Design review of the part built by this model. Coordinates are the model's own, in mm. Face numbers are marked on the shaded views. Coordinates: 2 decimals unless noted, no trailing zeros. Order: outer loops, then holes, each group sorted by start corner. A loop starts at its lowest first (then second) coordinate and runs counter-clockwise, first axis right, second up. Notation, with made-up numbers: M 35,-18.5 L 87,-18.5 A24 ccw 87,-2.5 Z; hole C 9.5,36 d7. An arc over 180 degrees is marked long. Answer as a JSON object with one key per item and string values.
from build123d import *

# Parameters (mm, degrees)
SKETCH1_R                = 25.4
BOSS_EXTRUDE1_DEPTH      = 127
BOSS_EXTRUDE2_REACH      = 202
BOSS_EXTRUDE2_END_RADIUS = 25.4
SKETCH3_R                = 12.7
SKETCH4_R                = 20
BOSS_EXTRUDE3_DEPTH      = 12.7
FILLET1_R                = 15.08


with BuildPart() as part:
    # Sketch1 → Boss-Extrude1 (new body)
    with BuildSketch(Plane(origin=(0, 0, 0), x_dir=(1, 0, 0), z_dir=(0, 1, 0))):
        with Locations(Location((0, 0, 0), (0, 0, 270))):
            Circle(SKETCH1_R)
    extrude(amount=BOSS_EXTRUDE1_DEPTH)

    # Boss-Extrude2: up to this cylinder (the profile starts outside it)
    boss_extrude2_end = Plane(origin=(0, 19.05, 0), z_dir=(0, -1, 0)) * Cylinder(BOSS_EXTRUDE2_END_RADIUS, 455.8, mode=Mode.PRIVATE)
    # Sketch3 → Boss-Extrude2 (add, up to the surface)
    with BuildSketch(Plane(origin=(127, 0, 0), x_dir=(0, 0, -1), z_dir=(1, 0, 0)), mode=Mode.PRIVATE) as boss_extrude2_sk1:
        with Locations((0, 19.05)):
            Circle(SKETCH3_R)
    boss_extrude2_tool1 = extrude(boss_extrude2_sk1.sketch, amount=-BOSS_EXTRUDE2_REACH, mode=Mode.PRIVATE) - boss_extrude2_end
    add(boss_extrude2_tool1.solids().sort_by_distance((127, 19.05, 0))[0])

    # Sketch4 → Boss-Extrude3 (add)
    with BuildSketch(Plane(origin=(127, 0, 0), x_dir=(0, 0, -1), z_dir=(1, 0, 0))):
        with Locations((0, 19.05)):
            Circle(SKETCH4_R)
    extrude(amount=BOSS_EXTRUDE3_DEPTH)

    # Fillet1
    # the kernel refuses this fillet: 15.08 mm, written as the material it takes off along each edge
    with BuildSketch(Plane(origin=(139.7, 19.05, 0), x_dir=(0, 0, -1), z_dir=(0, -1, 0))) as fillet1_piece_1:
        with BuildLine():
            CenterArc((5.108996004, -15.08), FILLET1_R, 9.080670078, 80.919329922)
            Line((5.108996004, 0), (5.108996004, 0.3016))
            Line((5.108996004, 0.3016), (20, 0.3016))
            Line((20, 0.3016), (20.3016, 0))
            ThreePointArc((20.3016, 0), (20.3016, -6.35), (20.29782008, -12.6524))
            Line((20.29782008, -12.6524), (20, -12.7))
        make_face()
    revolve(axis=Axis((139.7, 19.05, 0), (1, 0, 0)), mode=Mode.SUBTRACT)


solid = part.part
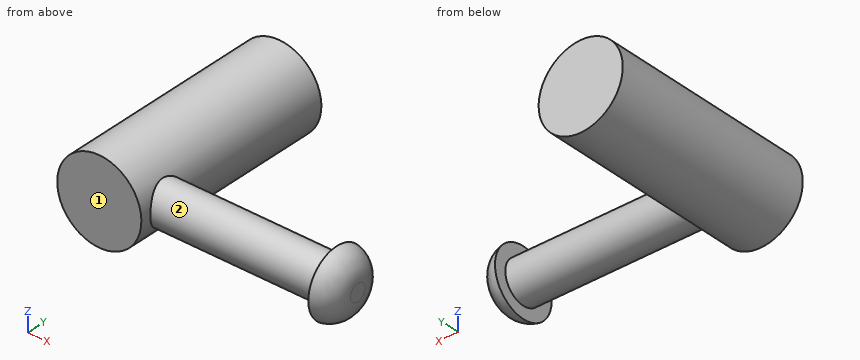
1) To check wall thickness, follow L1, parallel to X at y = 28, z = -12; L2, parallel to Y at x = 4, z = 11.5; L3, parallel to Z at x = -3.5, y = 98.5. State the ranges of each line that lie inside material, in increasing order.
Taken from the geometry:
{"L1": "x = -22.39 to 22.39, 127 to 136.03", "L2": "y = 0 to 127", "L3": "z = -25.16 to 25.16"}
2) Add section C-C (x = -10). State the section outline as (y, z) points.
Taken from the geometry:
{"outline": "M 0,-23.35 L 127,-23.35 L 127,23.35 L 0,23.35 Z"}
3) Mouldability with a two-part tool opening along X and no side actions: class the marked faces 1 and 2 as released by +X, released by -X, zero draft, split by the parting line, or undercut.
Taken from the geometry:
{"face 1": "zero draft", "face 2": "undercut"}
4) Insertion check: pin 1 Ø3 at (y, z) = (103, 19) entering from -X; pin 2 Ø10 at (y, z) = (74, -11.5) entering from -X; pin 3 Ø15 at (x, z) = (-8.5, 4.5) entering from -Y. Each pin has a flat end and moves straight along its axis. Give the tip position at first contact, or say it passes through.
Taken from the geometry:
{"pin 1": "stops at x = -18.41", "pin 2": "stops at x = -24.55", "pin 3": "stops at y = 0"}
5) Add section B-B (y = 110.5). State the section outline as (x, z) points.
Taken from the geometry:
{"outline": "C 0,0 d50.8"}
6) Add section A-A (x = 68). State the section outline as (y, z) points.
Taken from the geometry:
{"outline": "C 19.05,0 d25.4"}
